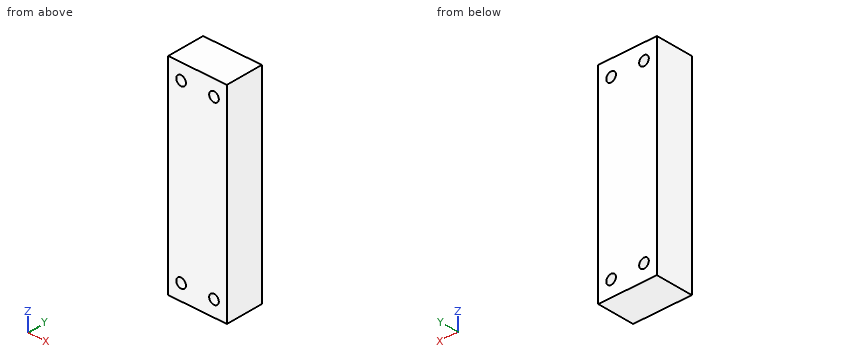
Autodesk Inventor part; units mm, degrees
ref_plane "YZ Plane" through (0, 0, 0) normal (1, 0, 0) x (0, 1, 0)
ref_plane "XZ Plane" through (0, 0, 0) normal (0, 1, 0) x (-1, 0, 0)
ref_plane "XY Plane" through (0, 0, 0) normal (0, 0, 1) x (1, 0, 0)
sketch "Sketch2" plane through (0, 0, 0) normal (0, 0, 1) x (1, 0, 0)
  line L0 (-25, 16) -> (25, 16)
  line L1 (25, 16) -> (25, -16)
  line L2 (25, -16) -> (-25, -16)
  line L3 (-25, -16) -> (-25, 16)
  line L4 (-25, 16) -> (25, -16) construction
  line L5 (25, 16) -> (-25, -16) construction
  point P0 (0, 0)
  dimension "d4" = 32
  dimension "d5" = 50
extrude "Extrusion1" add sketch "Sketch2" along normal mid plane 176
sketch "Sketch5" plane through (0, 0, -88) normal (0, 0, -1) x (-1, 0, 0)
  line L0 (-14, 0) -> (-25, 0) construction
  line L1 (-25, -16) -> (-25, 16)
  line L2 (14, 0) -> (25, 0) construction
  line L3 (25, 16) -> (25, -16)
  line L4 (-25, 0) -> (25, 0) construction
  point P0 (0, 0)
  dimension "d14" = 28
sketch "Sketch6" plane through (-25, -16, -88) normal (0, -1, 0) x (1, 0, 0)
  point P0 (25, 88)
sketch "Sketch9" plane through (-25, -16, 88) normal (0, -1, 0) x (1, 0, 0)
  line L0 (0, 0) -> (50, 0)
  line L1 (39, 0) -> (39, -176) construction
  line L2 (0, -176) -> (50, -176)
  line L3 (50, -176) -> (0, -176) construction
  line L4 (39, -13.5) -> (50, -13.5) construction
  line L5 (50, -176) -> (50, 0) construction
  line L6 (11, -13.5) -> (0, -13.5) construction
  line L7 (0, 0) -> (0, -176) construction
  line L8 (11, -13.5) -> (11, 0)
  line L9 (11, -162.5) -> (0, -162.5) construction
  line L10 (11, -162.5) -> (11, -176) construction
  point P0 (25, -88)
  point P1 (39, -162.5)
  dimension "d36" = 28
  dimension "d37" = 28
  dimension "d38" = 149
hole "Hole3" at (14, -16, 74.5) at (-14, -16, 74.5) at (14, -16, -74.5) at (-14, -16, -74.5) direction (0, 1, 0) diameter 8.2 end through all
properties part number "13042026-05"
Design review of the part built by this model. Coordinates are the model's own, in mm. Round coordinates to 2 decimals unless told otherwise and drop trailing zeros. Write each loop counter-clockwise with the first axis right and the second up, starting at its lowest first coordinate (ties: lowest second). Pieces come first, ordered by that corner, then holes. Notation, with made-up numbers: (28, -33) -> (63, -33) arc R26 cw to (63, 3) -> close; hole circle Ø11 at (70.25, -19.5). An arc over 180 degrees is marked (long way). Write item = value, one per line. Start each with the question number.
1) Take a section at C-C, the plane z = 74.5. State the section outline as (x, y) points.
2) Wall thickness on probe 1 along Z at (x, y) = (14, -1.5); probe 2 along X at (y, z) = (-5, 74.5): over which ranges is each line inside the solid? List them lowest first. Write a range as from..to.
3) Take a section at B-B, the plane y = -11. State the section outline as (x, z) points.
4) Take a section at A-A, the plane x = 14. State the section outline as (y, z) points, plus the area to 3 significant figures.
Results list:
q1.outline = (-25, -16) -> (-18.1, -16) -> (-18.1, 16) -> (-25, 16) -> close; (-9.9, -16) -> (9.9, -16) -> (9.9, 16) -> (-9.9, 16) -> close; (18.1, -16) -> (25, -16) -> (25, 16) -> (18.1, 16) -> close
q2.probe_1 = -88..-78.6, -70.4..70.4, 78.6..88
q2.probe_2 = -25..-18.1, -9.9..9.9, 18.1..25
q3.outline = (-25, -88) -> (25, -88) -> (25, 88) -> (-25, 88) -> close; hole circle Ø8.2 at (-14, -74.5); hole circle Ø8.2 at (-14, 74.5); hole circle Ø8.2 at (14, -74.5); hole circle Ø8.2 at (14, 74.5)
q4.outline = (-16, -88) -> (16, -88) -> (16, -78.6) -> (-16, -78.6) -> close; (-16, -70.4) -> (16, -70.4) -> (16, 70.4) -> (-16, 70.4) -> close; (-16, 78.6) -> (16, 78.6) -> (16, 88) -> (-16, 88) -> close
q4.area = 5,110 mm²
